```python
from build123d import *

# Parameters (mm, degrees)
F1_DEPTH = 25.4


with BuildPart() as f1:
    # F0 (on Front) → F1 (new body)
    with BuildSketch(Plane.XZ):
        with BuildLine():
            ThreePointArc((48.680444, -2.920995), (48.746106, -1.461153), (48.768, 0))
            ThreePointArc((48.768, 0), (48.546173, 4.646173), (47.88271, 9.250078))
            ThreePointArc((47.88271, 9.250078), (46.733738, 13.938277), (45.126937, 18.489927))
            ThreePointArc((45.126937, 18.489927), (42.460467, 23.98805), (39.127372, 29.109562))
            ThreePointArc((39.127372, 29.109562), (36.058052, 32.834962), (32.635486, 36.238693))
            ThreePointArc((32.635486, 36.238693), (27.847534, 40.035392), (22.622379, 43.203539))
            ThreePointArc((22.622379, 43.203539), (18.240626, 45.228281), (13.680177, 46.809941))
            ThreePointArc((13.680177, 46.809941), (7.719056, 48.153235), (1.636746, 48.740526))
            ThreePointArc((1.636746, 48.740526), (-3.18958, 48.663584), (-7.984658, 48.109906))
            ThreePointArc((-7.984658, 48.109906), (-13.938277, 46.733738), (-19.673065, 44.623854))
            ThreePointArc((-19.673065, 44.623854), (-23.98805, 42.460467), (-28.068034, 39.881114))
            ThreePointArc((-28.068034, 39.881114), (-32.834962, 36.058052), (-37.086384, 31.66888))
            ThreePointArc((-37.086384, 31.66888), (-40.035392, 27.847534), (-42.592192, 23.753379))
            ThreePointArc((-42.592192, 23.753379), (-45.228281, 18.240626), (-47.154289, 12.441496))
            ThreePointArc((-47.154289, 12.441496), (-48.153235, 7.719056), (-48.680444, 2.920995))
            ThreePointArc((-48.680444, 2.920995), (-48.663584, -3.18958), (-47.88271, -9.250078))
            ThreePointArc((-47.88271, -9.250078), (-46.733738, -13.938277), (-45.126937, -18.489927))
            ThreePointArc((-45.126937, -18.489927), (-42.460467, -23.98805), (-39.127372, -29.109562))
            ThreePointArc((-39.127372, -29.109562), (-36.058052, -32.834962), (-32.635486, -36.238693))
            ThreePointArc((-32.635486, -36.238693), (-27.847534, -40.035392), (-22.622379, -43.203539))
            ThreePointArc((-22.622379, -43.203539), (-18.240626, -45.228281), (-13.680177, -46.809941))
            ThreePointArc((-13.680177, -46.809941), (-7.719056, -48.153235), (-1.636746, -48.740526))
            ThreePointArc((-1.636746, -48.740526), (3.18958, -48.663584), (7.984658, -48.109906))
            ThreePointArc((7.984658, -48.109906), (13.938277, -46.733738), (19.673065, -44.623854))
            ThreePointArc((19.673065, -44.623854), (23.98805, -42.460467), (28.068034, -39.881114))
            ThreePointArc((28.068034, -39.881114), (32.834962, -36.058052), (37.086384, -31.66888))
            ThreePointArc((37.086384, -31.66888), (40.035392, -27.847534), (42.592192, -23.753379))
            ThreePointArc((42.592192, -23.753379), (45.228281, -18.240626), (47.154289, -12.441496))
            ThreePointArc((47.154289, -12.441496), (48.153235, -7.719056), (48.680444, -2.920995))
        make_face()
        with BuildLine():
            ThreePointArc((-48.680444, 2.920995), (-48.153235, 7.719056), (-47.154289, 12.441496))
            ThreePointArc((-47.154289, 12.441496), (-52.152725, 13.171914), (-57.20292, 13.056193))
            ThreePointArc((-57.20292, 13.056193), (-59.960814, 12.434145), (-62.504457, 11.200127))
            ThreePointArc((-62.504457, 11.200127), (-62.699524, 10.050854), (-62.873461, 8.898193))
            ThreePointArc((-62.873461, 8.898193), (-60.842988, 6.930936), (-58.417717, 5.478016))
            ThreePointArc((-58.417717, 5.478016), (-53.656736, 3.789545), (-48.680444, 2.920995))
        make_face()
        with BuildLine():
            ThreePointArc((-42.592192, 23.753379), (-40.035392, 27.847534), (-37.086384, 31.66888))
            ThreePointArc((-37.086384, 31.66888), (-41.272902, 34.495704), (-45.87318, 36.582641))
            ThreePointArc((-45.87318, 36.582641), (-48.627853, 37.218799), (-51.455017, 37.210634))
            ThreePointArc((-51.455017, 37.210634), (-52.129417, 36.25981), (-52.78625, 35.296768))
            ThreePointArc((-52.78625, 35.296768), (-51.810418, 32.643341), (-50.255722, 30.28202))
            ThreePointArc((-50.255722, 30.28202), (-46.698827, 26.695048), (-42.592192, 23.753379))
        make_face()
        with BuildLine():
            ThreePointArc((-28.068034, 39.881114), (-23.98805, 42.460467), (-19.673065, 44.623854))
            ThreePointArc((-19.673065, 44.623854), (-22.218475, 48.987196), (-25.457695, 52.863447))
            ThreePointArc((-25.457695, 52.863447), (-27.66355, 54.631814), (-30.214279, 55.851118))
            ThreePointArc((-30.214279, 55.851118), (-31.23444, 55.287067), (-32.244075, 54.704384))
            ThreePointArc((-32.244075, 54.704384), (-32.516159, 51.890332), (-32.139965, 49.088297))
            ThreePointArc((-32.139965, 49.088297), (-30.491642, 44.313269), (-28.068034, 39.881114))
        make_face()
        with BuildLine():
            ThreePointArc((-7.984658, 48.109906), (-3.18958, 48.663584), (1.636746, 48.740526))
            ThreePointArc((1.636746, 48.740526), (1.236594, 53.776174), (0, 58.674))
            ThreePointArc((0, 58.674), (-1.220142, 61.224328), (-2.989233, 63.429603))
            ThreePointArc((-2.989233, 63.429603), (-4.153099, 63.364042), (-5.315565, 63.277127))
            ThreePointArc((-5.315565, 63.277127), (-6.781675, 60.859806), (-7.658494, 58.172036))
            ThreePointArc((-7.658494, 58.172036), (-8.245214, 53.154703), (-7.984658, 48.109906))
        make_face()
        with BuildLine():
            ThreePointArc((13.680177, 46.809941), (18.240626, 45.228281), (22.622379, 43.203539))
            ThreePointArc((22.622379, 43.203539), (24.44674, 47.91412), (25.457695, 52.863447))
            ThreePointArc((25.457695, 52.863447), (25.464931, 55.690613), (24.827867, 58.445077))
            ThreePointArc((24.827867, 58.445077), (23.750815, 58.890991), (22.665758, 59.317058))
            ThreePointArc((22.665758, 59.317058), (20.296002, 57.775249), (18.339836, 55.734089))
            ThreePointArc((18.339836, 55.734089), (15.634281, 51.468197), (13.680177, 46.809941))
        make_face()
    extrude(amount=F1_DEPTH)


solid = f1.part
```
Can you work these out from the model? Positions are in its coordinate system, mm. A direction names the side the tool comes from. Round coordinates to 2 decimals unless told otherwise and drop trailing zeros. Loops run counter-clockwise (first coordinate to the right, second up) from the corner with the lowest first, then second, coordinate; pieces in that order, holes last. Notation, with made-up numbers: M -1.5,-8.5 L 4.5,-8.5 A12 ccw 4.5,-0.5 Z; hole C 87.25,74.25 d4. An arc over 180 degrees is marked long. Write item = value, one per line. Start each with the question number.
(1) I need wall thicknesses on line 1 along Z through (x, y) = (-3, -6); line 2 along X through (y, z) = (-18.25, 35); line 3 along X through (y, z) = (-14.5, 57.5). Which ranges of each line are inside material? Lowest first, please.
(2) Which directions (+Z, -Z, +X, -X, +Y, -Y) give clear straight access to the entire face, cutting with the end or side of a thin tool? Please do faces 1 (the face through (-51.83, -12.52, 32.68)), 2 (the face through (-27.63, -12.52, 54.61)), 3 (the face through (25.47, -12.52, 55.65)).
(3) I'm going to push flat-ended pins straight in: P1, Ø4, axis at x = -19.5, y = -16.5, coming from the -Z side; P2, Ø10, axis at x = -7.5, y = -22.5, coming from the -Z side; P3, Ø2, axis at x = -33.5, y = -8.5, coming from the -Z side. Where does each tip first touch, or does it pass through?
(4) Suppose I cut it at B-B on z = -14. Write out the boundary of the cut face in (x, y).
(5) Suppose I cut it at A-A on z = -26.5. Write out the boundary of the cut face in (x, y), plus the area to 3 significant figures.
(6) If we mould it in two halves opening along Z, with no side actions, what happens to faces 4 (the face through (45.196, -12.522, -18.32)), 5 (the face through (27.9, -12.5, 40)), 6 (the face through (36.104, -12.522, 32.785))? For each: released by +Z, released by -Z, zero draft, split by the parting line, or undercut.
Answer block:
q1.line_1 = -48.68 to 63.43
q1.line_2 = -52.71 to -42.21, -33.96 to 33.96
q1.line_3 = -7.79 to 0.38, 19.98 to 25.12
q2.face_1 = -X, +Y, -Y
q2.face_2 = +Z, +Y, -Y
q2.face_3 = +X, +Y, -Y
q3.P1 = -45.52
q3.P2 = -48.7
q3.P3 = -36.36
q4.outline = M -46.72,-25.4 L 46.72,-25.4 L 46.72,0 L -46.72,0 Z
q5.outline = M -40.94,-25.4 L 40.94,-25.4 L 40.94,0 L -40.94,0 Z
q5.area = 2,080 mm²
q6.face_4 = released by -Z
q6.face_5 = undercut
q6.face_6 = released by +Z
